Work out the finished part from the listing and answer in its coordinate system (mm). Coordinates: 2 decimals unless noted, no trailing zeros. Loops run counter-clockwise (first coordinate to the right, second up) from the corner with the lowest first, then second, coordinate; pieces in that order, holes last. Notation, with made-up numbers: (55, 40) -> (67, 40) arc R31 ccw to (67, 78) -> close; hole circle Ø9 at (49, -10.75). An arc over 180 degrees is marked (long way). Use a Markdown table: item, result.
from build123d import *

# Parameters (mm, degrees)
BOSS_EXTRUDE1_DEPTH = 5


with BuildPart() as part:
    # Sketch1 → Boss-Extrude1 (new body)
    with BuildSketch(Plane.XY):
        Polygon((-8, 0), (0, 0), (0, -198), (2, -198), (2, 2), (-8, 2), align=None)
    extrude(amount=BOSS_EXTRUDE1_DEPTH)

    # Sketch3 → CSK for M2 Flat Head Machine Screw1 (revolve, cut)
    with BuildSketch(Plane(origin=(2, -78, 2.5), x_dir=(0, 0, -1), z_dir=(0, 1, 0))):
        Polygon((0, 0), (0, 2), (1.1, 2), (1.1, 1.1), (2.2, 0), align=None)
    revolve(axis=Axis((8.35, -78, 2.5), (-1, 0, 0)), mode=Mode.SUBTRACT)


solid = part.part
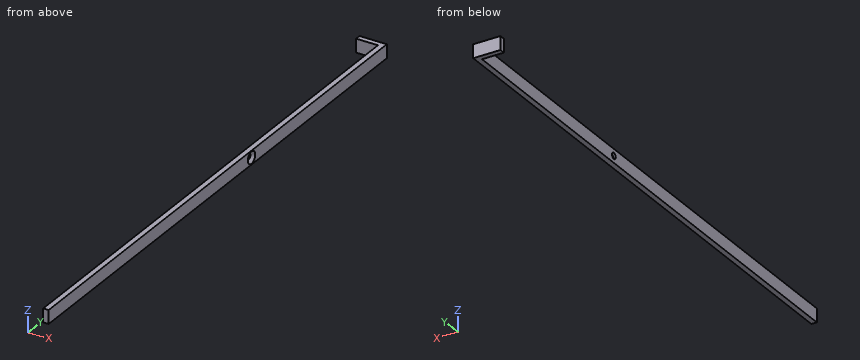
Q1. Given pin 1 Ø3 at (y, z) = (-115, 1) entering from -X; pin 2 Ø2 at (x, z) = (-6, 1) entering from -Y, each flat-ended and moving along its own axis, determine where each tip first touches the part or whether it passes through.
Solved:
| item | result |
|---|---|
| pin 1 | x = 0 |
| pin 2 | y = 0 |
Q2. Consider line 1 (Z direction, x = 0.6, y = -78); line 2 (Y direction, x = 0.75, z = 2.5); line 3 (Y direction, x = -2.25, z = 2.6). Determine where each line is inside the solid, lowest interval first. Write a range as [from, to].
Solved:
| item | result |
|---|---|
| line 1 | [0, 1.4], [3.6, 5] |
| line 2 | [-198, -79.1], [-76.9, 2] |
| line 3 | [0, 2] |
Q3. Section A-A on z = 2.5 is taken. Determine the outline of the cut face in (x, y).
Solved:
| item | result |
|---|---|
| outline | (-8, 0) -> (0, 0) -> (0, -76.9) -> (0.9, -76.9) -> (2, -75.8) -> (2, 2) -> (-8, 2) -> close; (0, -198) -> (2, -198) -> (2, -80.2) -> (0.9, -79.1) -> (0, -79.1) -> close |
Q4. Section B-B on y = -170.5 is taken. Determine the outline of the cut face in (x, z), and give its area (3 significant figures).
Solved:
| item | result |
|---|---|
| outline | (0, 0) -> (2, 0) -> (2, 5) -> (0, 5) -> close |
| area | 10.0 mm² |
